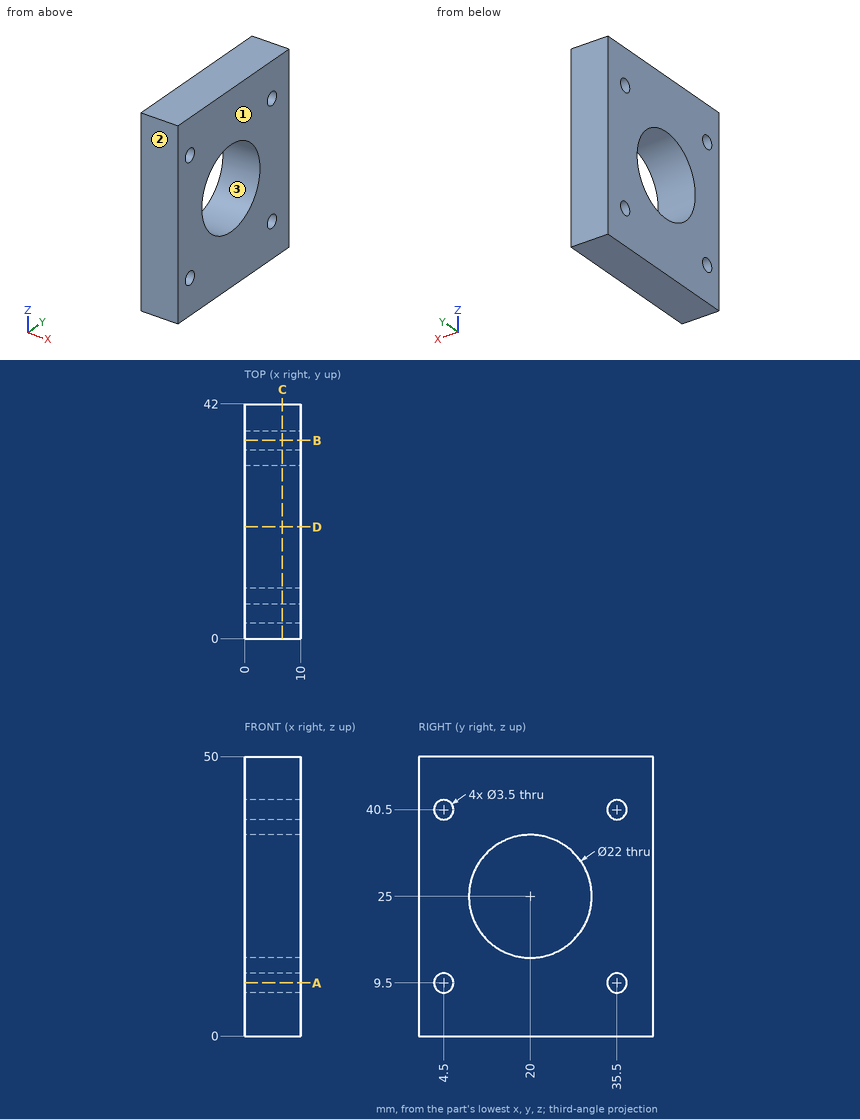
Geometry check sheet. Reference: drawing and pictorial views, mm from the part's lowest x, y, z. Round coordinates to 2 decimals unless told otherwise and drop trailing zeros. Order: outer loops, then holes, each group sorted by start corner. A loop starts at its lowest first (then second) coordinate and runs counter-clockwise, first axis right, second up. Notation, with made-up numbers: (25.5, 56) - (52.5, 56) arc R19 cw to (52.5, 63) - close; hole circle Ø4 at (-29.75, 79). An arc over 180 degrees is marked (long way). Use a Markdown table: item, result. Add a question column.
1) Section check A-A (z = 9.5). Record the cut outline in (x, y).
2) Section check D-D (y = 20). Record the cut outline in (x, z).
3) Mould release check, pull along Y, two halves, no side actions. Record for the marked faces 1, 2 and 3: released by +Y, released by -Y, zero draft, split by the parting line, or undercut.
4) Thickness scan on line 1 along Z through (x, y) = (6, 4.5); line 2 along Z through (x, y) = (4, 3); line 3 along Y through (x, z) = (8.25, 42). Record the ranges inside material, lowest first.
5) Section check B-B (y = 35.5). Record the cut outline in (x, z).
6) Section check C-C (x = 6.75). Record the cut outline in (y, z), then the cut area to 3 significant figures.
Established:
| question | item | result |
|---|---|---|
| 1 | outline | (0, 0) - (10, 0) - (10, 2.75) - (0, 2.75) - close; (0, 6.25) - (10, 6.25) - (10, 33.75) - (0, 33.75) - close; (0, 37.25) - (10, 37.25) - (10, 42) - (0, 42) - close |
| 2 | outline | (0, 0) - (10, 0) - (10, 14) - (0, 14) - close; (0, 36) - (10, 36) - (10, 50) - (0, 50) - close |
| 3 | face 1 | zero draft |
| 3 | face 2 | released by -Y |
| 3 | face 3 | undercut |
| 4 | line 1 | 0 to 7.75, 11.25 to 38.75, 42.25 to 50 |
| 4 | line 2 | 0 to 8.6, 10.4 to 39.6, 41.4 to 50 |
| 4 | line 3 | 0 to 3.6, 5.4 to 34.6, 36.4 to 42 |
| 5 | outline | (0, 0) - (10, 0) - (10, 7.75) - (0, 7.75) - close; (0, 11.25) - (10, 11.25) - (10, 38.75) - (0, 38.75) - close; (0, 42.25) - (10, 42.25) - (10, 50) - (0, 50) - close |
| 6 | outline | (0, 0) - (42, 0) - (42, 50) - (0, 50) - close; hole circle Ø3.5 at (4.5, 9.5); hole circle Ø3.5 at (4.5, 40.5); hole circle Ø22 at (20, 25); hole circle Ø3.5 at (35.5, 9.5); hole circle Ø3.5 at (35.5, 40.5) |
| 6 | area | 1,680 mm2 |
